Geometry: final body of the model. Coordinates: model frame, mm. A direction names the side the tool comes from. Coordinates: 2 decimals unless noted, no trailing zeros. Order: outer loops, then holes, each group sorted by start corner. A loop starts at its lowest first (then second) coordinate and runs counter-clockwise, first axis right, second up. Notation, with made-up numbers: (-7, -22.5) - (22, -22.5) arc R12 ccw to (22, -6.5) - close; hole circle Ø10 at (62.25, 78). An arc over 180 degrees is marked (long way). Use a Markdown table: item, result. Add a question column.
```python
from build123d import *

# Parameters (mm, degrees)
SKETCH1_R                 = 20
BOSS_EXTRUDE1_DEPTH       = 25
M5X0_8_TAPPED_HOLE1_D     = 4.2
M5X0_8_TAPPED_HOLE1_DEPTH = 18.7381927
M5X0_8_TAPPED_HOLE1_TIP   = 1.2618073


with BuildPart() as part:
    # Sketch1 → Boss-Extrude1 (new body, symmetric)
    with BuildSketch(Plane(origin=(0, 0, 0), x_dir=(1, 0, 0), z_dir=(0, 1, 0))):
        Circle(SKETCH1_R)
    extrude(amount=BOSS_EXTRUDE1_DEPTH, both=True)

    # M5x0.8 Tapped Hole1
    with Locations(Plane(origin=(0, 25, -12), x_dir=(0, 0, 1), z_dir=(0, 1, 0))):
        with Locations((0, 0), (12, 12), (24, 0), (12, -12)):
            Hole(M5X0_8_TAPPED_HOLE1_D / 2, depth=M5X0_8_TAPPED_HOLE1_DEPTH)
            with Locations((0, 0, -(M5X0_8_TAPPED_HOLE1_DEPTH + M5X0_8_TAPPED_HOLE1_TIP / 2))):  # 118° drill point
                Cone(0, M5X0_8_TAPPED_HOLE1_D / 2, M5X0_8_TAPPED_HOLE1_TIP, mode=Mode.SUBTRACT)


solid = part.part
```
1) Section B-B (x = 16). Return loops of the section in (y, z), then the cut area to 3 significant figures.
2) Ray query, line 1 along X through (y, z) = (11, 0); line 2 along Z through (x, y) = (-12, 14). Return the intervals inside material, ascending.
3) Set-up query: faces 1 (the face through (0, -25, 0)), 2 (the face through (0.09, 15.5, -9.9)). Return all of +Z, -Z, +X, -X, +Y, -Y with unobstructed straight access to the full face (end or side cutting, diameter ignored); none if empty.
4) Section C-C (y = -9). Return loops of the section in (x, z), then the cut area to 3 significant figures.
5) Section A-A (y = 10.5). Return loops of the section in (x, z).
6) Draft query along Z for faces 3 (the face through (-4.336, 0.35, 19.524)), 4 (the face through (0, 25, 0)), 5 (the face through (14.082, 15.5, 0.273)). Return one class per face: pulls with the +Z half, pulls with the -Z half, needs draft (parallel to the pull), parting line crosses it, or undercut.
7) Pin query (flat end, axial travel): pin 1 (10 mm diameter, centred on y = 17, z = 16, fed in from -X); pin 2 (12 mm diameter, centred on y = -2.5, z = -15, fed in from -X); pin 3 (1 mm diameter, centred on x = 6.5, y = -17.5, fed in from +Z). Return the tip coordinate at first contact, or that it passes through.
8) Section D-D (z = -16). Return loops of the section in (x, y), then the cut area to 3 significant figures.
Values follow:
| question | item | result |
|---|---|---|
| 1 | outline | (-25, -12) - (25, -12) - (25, 12) - (-25, 12) - close |
| 1 | area | 1,200 mm² |
| 2 | line 1 | x = -20 to -14.1, -9.9 to 9.9, 14.1 to 20 |
| 2 | line 2 | z = -16 to -2.1, 2.1 to 16 |
| 3 | face 1 | +Z, -Z, +X, -X, -Y |
| 3 | face 2 | +Y |
| 4 | outline | circle Ø40 at (0, 0) |
| 4 | area | 1,260 mm² |
| 5 | outline | circle Ø40 at (0, 0); hole circle Ø4.2 at (-12, 0); hole circle Ø4.2 at (0, -12); hole circle Ø4.2 at (0, 12); hole circle Ø4.2 at (12, 0) |
| 6 | face 3 | parting line crosses it |
| 6 | face 4 | needs draft |
| 6 | face 5 | undercut |
| 7 | pin 1 | stops at x = -16.7 |
| 7 | pin 2 | stops at x = -17.86 |
| 7 | pin 3 | stops at z = 19.08 |
| 8 | outline | (-12, -25) - (12, -25) - (12, 25) - (-12, 25) - close |
| 8 | area | 1,200 mm² |
